Could you check a few things on this model? Use its own coordinates, in mm. Give positions to 0.01 mm unless a question says otherwise; leave off trailing zeros. Loops run counter-clockwise (first coordinate to the right, second up) from the corner with the lowest first, then second, coordinate; pieces in that order, holes last. Notation, with made-up numbers: M 80.25,37.5 L 120.25,37.5 A17 cw 120.25,47.5 Z; hole C -17,12.25 d6. An arc over 180 degrees is marked long. Use a Markdown table: item, result. Add a question column.
1) Will this pin go through, and if not, where does the flat tip stop? pin 1 Ø3 at (x, y) = (-37.5, 20.625) entering from +Z.
2) Suppose I cut it at A-A on x = 37.5. List the corners of the cut face in (y, z) for me (3 decimals).
3) We'd pull the mould along X, two halves only. Please class faces 1 (the cylindrical face through (41.43, 23.4, -23.14)), 2 (the cylindrical face through (36.51, 19.86, -22.75)), 3 (the flat face through (-1, 0, -23.385)): +X half, -X half, draft (parallel to the pull), parting line (faces both ways), or undercut.
4) If I drill on line 1 along Y through (x, z) = (37.5, -22.9) (3 decimals); line 2 along Y through (x, z) = (-37.5, -22.5) (3 decimals); line 3 along X through (y, z) = (13.5, -22.75), over which ranges is the centre line in solid material (lowest first)? Write a range as [from, to].
```python
from build123d import *

# Parameters (mm, degrees)
SKETCH_2_R      = 1.25
EXTRUDE_1_DEPTH = 2
FILLET_1_R      = 1.5
CHAMFER_1_SIZE  = 0.5
CHAMFER_1_SIZE2 = 0.714074003


with BuildPart() as part:
    # 草图2 → 凸台-拉伸1 (new body)
    with BuildSketch(Plane.XY.offset(-23.385365979)):
        with BuildLine():
            Line((-42, 22), (-42, -22))
            ThreePointArc((-42, -22), (-41.414213562, -23.414213562), (-40, -24))
            Line((-40, -24), (40, -24))
            ThreePointArc((40, -24), (41.414213562, -23.414213562), (42, -22))
            Line((42, -22), (42, 22))
            ThreePointArc((42, 22), (41.414213562, 23.414213562), (40, 24))
            Line((40, 24), (-40, 24))
            ThreePointArc((-40, 24), (-41.414213562, 23.414213562), (-42, 22))
        make_face()
        with Locations((37.5, -20.625)):
            Circle(SKETCH_2_R, mode=Mode.SUBTRACT)
        with Locations((-37.5, -20.625)):
            Circle(SKETCH_2_R, mode=Mode.SUBTRACT)
        with Locations((37.5, 20.625)):
            Circle(SKETCH_2_R, mode=Mode.SUBTRACT)
        with Locations((-37.5, 20.625)):
            Circle(SKETCH_2_R, mode=Mode.SUBTRACT)
    extrude(amount=EXTRUDE_1_DEPTH)

    # 圆角1
    fillet_1_edges = [part.edges().sort_by_distance(p)[0] for p in [
        (-41.414213562, -23.414213562, -21.385365979),
        (0, -24, -21.385365979),
        (41.414213562, -23.414213562, -21.385365979),
        (42, 0, -21.385365979),
        (41.414213562, 23.414213562, -21.385365979),
        (0, 24, -21.385365979),
        (-41.414213562, 23.414213562, -21.385365979),
        (-42, 0, -21.385365979),
    ]]
    fillet(fillet_1_edges, radius=FILLET_1_R)

    # 倒角1
    chamfer_1_edges = [part.edges().sort_by_distance(p)[0] for p in [
        (36.25, -20.625, -21.385365979),
        (-38.75, -20.625, -21.385365979),
        (36.25, 20.625, -21.385365979),
        (-38.75, 20.625, -21.385365979),
    ]]
    chamfer_1_side = [part.faces().sort_by_distance(p)[0] for p in [
        (0, 0, -21.385365979),
    ]]
    chamfer(chamfer_1_edges, length=CHAMFER_1_SIZE, length2=CHAMFER_1_SIZE2, reference=chamfer_1_side[0])


solid = part.part
```
Answer block:
| question | item | result |
|---|---|---|
| 1 | pin 1 | stops at z = -21.74 |
| 2 | outline | M -24,-23.385 L -21.875,-23.385 L -21.875,-22.099 L -22.375,-21.385 L -22.5,-21.385 A1.5 ccw -24,-22.885 Z; M -19.375,-23.385 L 19.375,-23.385 L 19.375,-22.099 L 18.875,-21.385 L -18.875,-21.385 L -19.375,-22.099 Z; M 21.875,-23.385 L 24,-23.385 L 24,-22.885 A1.5 ccw 22.5,-21.385 L 22.375,-21.385 L 21.875,-22.099 Z |
| 3 | face 1 | +X half |
| 3 | face 2 | undercut |
| 3 | face 3 | draft |
| 4 | line 1 | y = [-24, -21.875], [-19.375, 19.375], [21.875, 24] |
| 4 | line 2 | y = [-23.95, -21.875], [-19.375, 19.375], [21.875, 23.95] |
| 4 | line 3 | x = [-41.99, 41.99] |
